Here's how the part is built. I have some questions about the finished solid (model axes, mm). Coordinates: 2 decimals unless noted, no trailing zeros. Order: outer loops, then holes, each group sorted by start corner. A loop starts at its lowest first (then second) coordinate and runs counter-clockwise, first axis right, second up. Notation, with made-up numbers: (-17.5, 22) - (7.5, 22) arc R36 ccw to (7.5, 61) - close; hole circle Ø10 at (74.5, -21.5). An arc over 180 degrees is marked (long way). Answer as CSV lines item,"result". Start each with the question number.
Q1. For pin 1 Ø1.6 at (x, y) = (0, 15.2) entering from +Z, with a flat end and sliding along its axis, tell me the tip position at first contact or that it passes through.
Q2. Thinking about a two-plate mould opening in X: for faces 1 (the face through (-0.217, 14.224, -0.789)), 2 (the face through (0, 8, 0)), 3 (the face through (-0.13, 31.39, -0.79)), 4 (the face through (-7.415, 7, -1)), which applies, released by +X, released by -X, zero draft, split by the parting line, or undercut?
Q3. Suppose I cut it at B-B (x = 0). Please give me the cut outline in (y, z), then the cut area to 3 significant figures.
Q4. I need wall thicknesses on line 1 (Y direction, x = 0, z = -1); line 2 (X direction, y = 14.5, z = -1.3); line 3 (X direction, y = 29.5, z = -0.1). Which ranges of each line are inside material? Lowest first, please.
Q5. Suppose I cut it at A-A (y = -15.2). Please give me the cut outline in (x, z).
from build123d import *

# Parameters (mm, degrees)
F1_W     = 15.2
F1_H     = 60.76299
F2_DEPTH = 1.6
F0_R     = 1
F3_DEPTH = 25


with BuildPart() as f2:
    # F1 (on Top) → F2 (new body)
    with BuildSketch(Plane.XY):
        with Locations((0.184545, 7.447379)):
            Rectangle(F1_W, F1_H)
    extrude(amount=-F2_DEPTH)

    # F0 (on Top) → F3 (cut)
    with BuildSketch(Plane.XY):
        Circle(F0_R)
        with Locations((0, 15.2)):
            Circle(F0_R)
        with Locations((0, 30.4)):
            Circle(F0_R)
        with Locations((0, -15.2)):
            Circle(F0_R)
    extrude(amount=-F3_DEPTH, mode=Mode.SUBTRACT)


solid = f2.part
Here are the results:
1,pin 1,"passes through"
2,face 1,"undercut"
2,face 2,"zero draft"
2,face 3,"undercut"
2,face 4,"released by -X"
3,outline,"(-22.93, -1.6) - (-16.2, -1.6) - (-16.2, 0) - (-22.93, 0) - close; (-14.2, -1.6) - (-1, -1.6) - (-1, 0) - (-14.2, 0) - close; (1, -1.6) - (14.2, -1.6) - (14.2, 0) - (1, 0) - close; (16.2, -1.6) - (29.4, -1.6) - (29.4, 0) - (16.2, 0) - close; (31.4, -1.6) - (37.83, -1.6) - (37.83, 0) - (31.4, 0) - close"
3,area,"84.4 mm²"
4,line 1,"y = -22.93 to -16.2, -14.2 to -1, 1 to 14.2, 16.2 to 29.4, 31.4 to 37.83"
4,line 2,"x = -7.42 to -0.71, 0.71 to 7.78"
4,line 3,"x = -7.42 to -0.44, 0.44 to 7.78"
5,outline,"(-7.42, -1.6) - (-1, -1.6) - (-1, 0) - (-7.42, 0) - close; (1, -1.6) - (7.78, -1.6) - (7.78, 0) - (1, 0) - close"
